Design review of the part built by this model. Coordinates are the model's own, in mm. Face numbers are marked on the shaded views. A direction names the side the tool comes from. Give positions to 0.01 mm unless a question says otherwise; leave off trailing zeros. Write each loop counter-clockwise with the first axis right and the second up, starting at its lowest first coordinate (ties: lowest second). Pieces come first, ordered by that corner, then holes. Notation, with made-up numbers: (1.25, -4.5) -> (38.25, -4.5) arc R26 cw to (38.25, 19.5) -> close; hole circle Ø5 at (53, 54). An arc over 180 degrees is marked (long way). Answer as a JSON object with one key per item and string values.
```python
from build123d import *

# Parameters (mm, degrees)
PAD_DEPTH    = 5
SKETCH001_R  = 13
SKETCH001_W  = 70
SKETCH001_H  = 58
PAD001_DEPTH = 2
FILLET_R     = 6


with BuildPart() as part:
    # Sketch → Pad (new body)
    with BuildSketch(Plane.XY):
        with BuildLine():
            ThreePointArc((1.143406, 102.474844), (-10.692396, 51.363106), (0, 0))
            Line((0, 0), (143.6, 0))
            ThreePointArc((143.6, 0), (154.292396, 51.363106), (142.456594, 102.474844))
            ThreePointArc((142.456594, 102.474844), (127.887765, 118.897055), (106.8, 125))
            Line((36.8, 125), (106.8, 125))
            ThreePointArc((36.8, 125), (15.712235, 118.897055), (1.143406, 102.474844))
        make_face()
    extrude(amount=PAD_DEPTH)

    # Sketch001 (on Face8 of Pad) → Pad001 (join)
    with BuildSketch(Plane.XY.offset(5)):
        with Locations((29.414366, 96.303098)):
            Circle(SKETCH001_R)
        with BuildLine():
            Line((114.734451, 111.679694), (118.692177, 114.166539))
            ThreePointArc((123.648757, 113.608086), (121.268173, 114.754509), (118.692177, 114.166539))
            Line((123.648757, 113.608086), (129.257643, 107.9992))
            ThreePointArc((128.55737, 101.783892), (130.404067, 104.72293), (129.257643, 107.9992))
            Line((128.55737, 101.783892), (124.599644, 99.297046))
            ThreePointArc((119.643063, 99.8555), (122.023647, 98.709076), (124.599644, 99.297046))
            Line((119.643063, 99.8555), (114.034177, 105.464386))
            ThreePointArc((114.734451, 111.679694), (112.887754, 108.740656), (114.034177, 105.464386))
        make_face()
        with BuildLine():
            Line((100.409759, 98.017022), (103.874582, 101.481845))
            ThreePointArc((109.531436, 101.481845), (106.703009, 102.653418), (103.874582, 101.481845))
            Line((109.531436, 101.481845), (115.400423, 95.612859))
            ThreePointArc((115.400423, 89.956005), (116.571995, 92.784432), (115.400423, 95.612859))
            Line((115.400423, 89.956005), (111.935599, 86.491182))
            ThreePointArc((106.278745, 86.491182), (109.107172, 85.319609), (111.935599, 86.491182))
            Line((106.278745, 86.491182), (100.409759, 92.360168))
            ThreePointArc((100.409759, 98.017022), (99.238186, 95.188595), (100.409759, 92.360168))
        make_face()
        with BuildLine():
            Line((90.420412, 88.28179), (82.286178, 81.642193))
            ThreePointArc((82.286178, 81.642193), (80.902255, 77.715104), (83.758696, 74.68558))
            Line((83.758696, 74.68558), (94.367803, 71.779235))
            ThreePointArc((94.367803, 71.779235), (96.449132, 71.770511), (98.253083, 72.808665))
            Line((98.253083, 72.808665), (101.788617, 76.344199))
            ThreePointArc((101.788617, 76.344199), (102.96019, 79.172626), (101.788617, 82.001054))
            Line((101.788617, 82.001054), (95.778209, 88.011461))
            ThreePointArc((95.778209, 88.011461), (93.151347, 89.177952), (90.420412, 88.28179))
        make_face()
        with Locations((71.8, 29)):
            Rectangle(SKETCH001_W, SKETCH001_H)
    extrude(amount=PAD001_DEPTH)

    # Fillet
    fillet_edges = [part.edges().sort_by_distance(p)[0] for p in [
        (36.8, 58, 6),
        (106.8, 58, 6),
    ]]
    fillet(fillet_edges, radius=FILLET_R)


solid = part.part
```
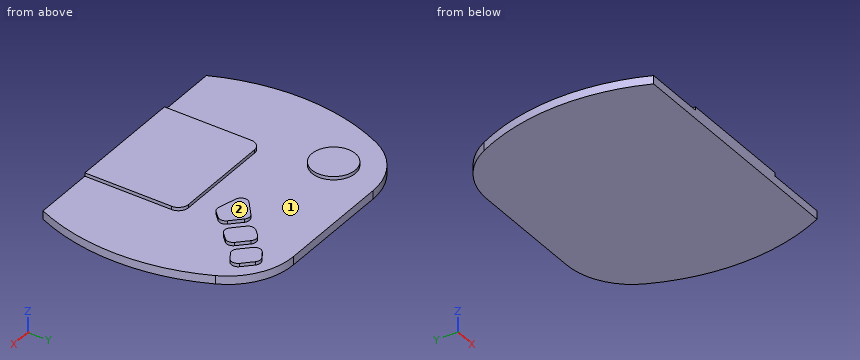
(1) For line 1 along X through (y, z) = (101.5, 5.75); line 2 along X through (y, z) = (10, 5.5); line 3 along Z through (x, y) = (111.5, 55), list the stretches that pass through material, from the lowest coordinate up.
Here are the results:
{"line 1": "x = 17.5 to 41.33, 103.89 to 109.51, 118 to 128.11", "line 2": "x = 36.8 to 106.8", "line 3": "z = 0 to 5"}
(2) We need section C-C, the plane z = 2.5. State the section outline as (x, y) points, then the cut area to 3 significant figures.
Here are the results:
{"outline": "(0, 0) -> (143.6, 0) arc R122.17 ccw to (142.46, 102.47) arc R39.48 ccw to (106.8, 125) -> (36.8, 125) arc R39.48 ccw to (1.14, 102.47) arc R122.17 ccw to start", "area": "18,900 mm²"}
(3) We need section D-D, the plane y = 67. State the section outline as (x, z) points, then the cut area to 3 significant figures.
Here are the results:
{"outline": "(-9.51, 0) -> (153.11, 0) -> (153.11, 5) -> (-9.51, 5) -> close", "area": "813 mm²"}
(4) We need section A-A, the plane y = 9. State the section outline as (x, z) points.
Here are the results:
{"outline": "(-3.61, 0) -> (147.21, 0) -> (147.21, 5) -> (106.8, 5) -> (106.8, 7) -> (36.8, 7) -> (36.8, 5) -> (-3.61, 5) -> close"}
(5) For the marked faces 1 and 2, list the 3-axis set-ups (+Z, -Z, +X, -X, +Y, -Y) from which the entire face can be reached by the end or side of a thin tool; tool diameter is ignored.
Here are the results:
{"face 1": "+Z", "face 2": "+Z, +X, -X, +Y, -Y"}
(6) Clearance check with a flat-ended pin moving along its axis: pin 1 (0.6 mm diameter, centred on y = 20, z = 5.5, fed in from +X). State where the tip first meets the part, or that it passes through.
Here are the results:
{"pin 1": "stops at x = 106.8"}
(7) We need section B-B, the plane x = 51.5. State the section outline as (y, z) points, then the cut area to 3 significant figures.
Here are the results:
{"outline": "(0, 0) -> (125, 0) -> (125, 5) -> (58, 5) -> (58, 7) -> (0, 7) -> close", "area": "741 mm²"}
